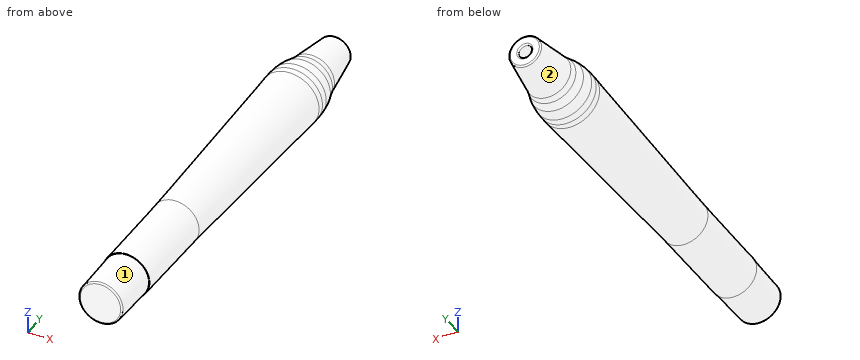
```python
from build123d import *

# Parameters (mm, degrees)
SKETCH_3_W = 9.44
SKETCH_3_H = 2.1
FILLET_1_R = 0.5


with BuildPart() as part:
    # 草图1 → 旋转1 (revolve)
    with BuildSketch(Plane.XY):
        Polygon((14.187329426, 38.64530146), (23.627329426, 38.64530146), (21.757329426, -29.909198757), (14.187329426, -29.909198757), align=None)
    revolve(axis=Axis((14.187329426, -29.909198757, 0), (0, 1, 0)))

    # 草图3 → 旋转2 (revolve)
    with BuildSketch(Plane.XY, mode=Mode.PRIVATE) as revolve_2_sk:
        with Locations((18.907329426, 39.69530146)):
            Rectangle(SKETCH_3_W, SKETCH_3_H)
    revolve(revolve_2_sk.sketch.rotate(Axis((14.187329426, 40.74530146, 0), (0, -1, 0)), 90), axis=Axis((14.187329426, 40.74530146, 0), (0, -1, 0)))

    # 草图5 → 旋转3 (revolve)
    with BuildSketch(Plane.XY, mode=Mode.PRIVATE) as revolve_3_sk:
        with BuildLine():
            Line((14.187329426, 40.74530146), (23.627329426, 40.74530146))
            Line((23.627329426, 40.74530146), (23.513107962, 43.195284059))
            ThreePointArc((23.513107962, 43.195284059), (23.30590626, 45.076327762), (22.863511042, 46.916312662))
            Line((22.863511042, 46.916312662), (21.973239823, 49.803743827))
            ThreePointArc((21.973239823, 49.803743827), (21.691526032, 50.850327778), (21.486119968, 51.914521827))
            Line((21.486119968, 51.914521827), (19.297329426, 65.96530146))
            Line((19.297329426, 65.96530146), (16.287329426, 65.96530146))
            Line((16.287329426, 65.96530146), (16.287329426, 60.46530146))
            Line((16.287329426, 60.46530146), (14.187329426, 60.46530146))
            Line((14.187329426, 60.46530146), (14.187329426, 40.74530146))
        make_face()
    revolve(revolve_3_sk.sketch.rotate(Axis((14.187329426, 60.46530146, 0), (0, -1, 0)), 180), axis=Axis((14.187329426, 60.46530146, 0), (0, -1, 0)))

    # 草图6 → 旋转4 (revolve)
    with BuildSketch(Plane.XY, mode=Mode.PRIVATE) as revolve_4_sk:
        Polygon((14.187329426, -29.909198757), (21.757329426, -29.909198757), (21.607329426, -59.478818302), (21.497329426, -59.478818302), (21.177329426, -75.027006041), (14.187329426, -75.027006041), (14.187329426, -59.478818302), align=None)
    revolve(revolve_4_sk.sketch.rotate(Axis((14.187329426, -59.478818302, 0), (0, 1, 0)), 270), axis=Axis((14.187329426, -59.478818302, 0), (0, 1, 0)))

    # 圆角1
    fillet_1_edges = [part.edges().sort_by_distance(p)[0] for p in [
        (16.287329426, 65.96530146, 0),
        (19.297329426, 65.96530146, 0),
        (14.187329426, -75.027006041, -6.99),
    ]]
    fillet(fillet_1_edges, radius=FILLET_1_R)


solid = part.part
```
Verification items for the finished model (mm, model axes). Face numbers are marked on the shaded views. A direction names the side the tool comes from. Coordinates: 2 decimals unless noted, no trailing zeros. Loops run counter-clockwise (first coordinate to the right, second up) from the corner with the lowest first, then second, coordinate; pieces in that order, holes last. Notation, with made-up numbers: (46.25, 0.25) - (55.25, 0.25) arc R18 cw to (55.25, 19.25) - close; hole circle Ø2 at (-35, 32). An arc over 180 degrees is marked (long way). Put each result on its own line as item: value.
Item 1: Section check A-A (y = -31.5). Enter the section's corners in (x, z), then the cut area to 3 significant figures.
Conclusion:
outline: circle Ø15.12 at (14.19, 0)
area: 180 mm2
Item 2: Gauge pin test, flat ends, axial feed: pin 1 Ø6 at (y, z) = (-37, -3.5) entering from +X; pin 2 Ø2 at (x, y) = (15, -21) entering from +Z; pin 3 Ø1 at (x, y) = (18, 22) entering from -Z. Record the tip position at first contact, or that the pin passes through.
Conclusion:
pin 1: stops at x = 21.71
pin 2: stops at z = 7.83
pin 3: stops at z = -8.35
Item 3: Section check B-B (y = -52.5). Enter the section's corners in (x, z).
Conclusion:
outline: circle Ø14.91 at (14.19, 0)
Item 4: Scan lines: line 1 along X through (y, z) = (-44.5, -1); line 2 along Z through (x, y) = (18, -2); line 3 along Y through (x, z) = (13.25, -1.5). Record each from-to range of solid material in increasing order.
Conclusion:
line 1: x = 6.76 to 21.62
line 2: z = -7.41 to 7.41
line 3: y = -75.03 to 60.47
Item 5: Set-up check for the marked faces 1 and 2: record each of +Z, -Z, +X, -X, +Y, -Y from which the full face is reachable in a straight line by a thin tool's end or side.
Conclusion:
face 1: -Y
face 2: +Y
